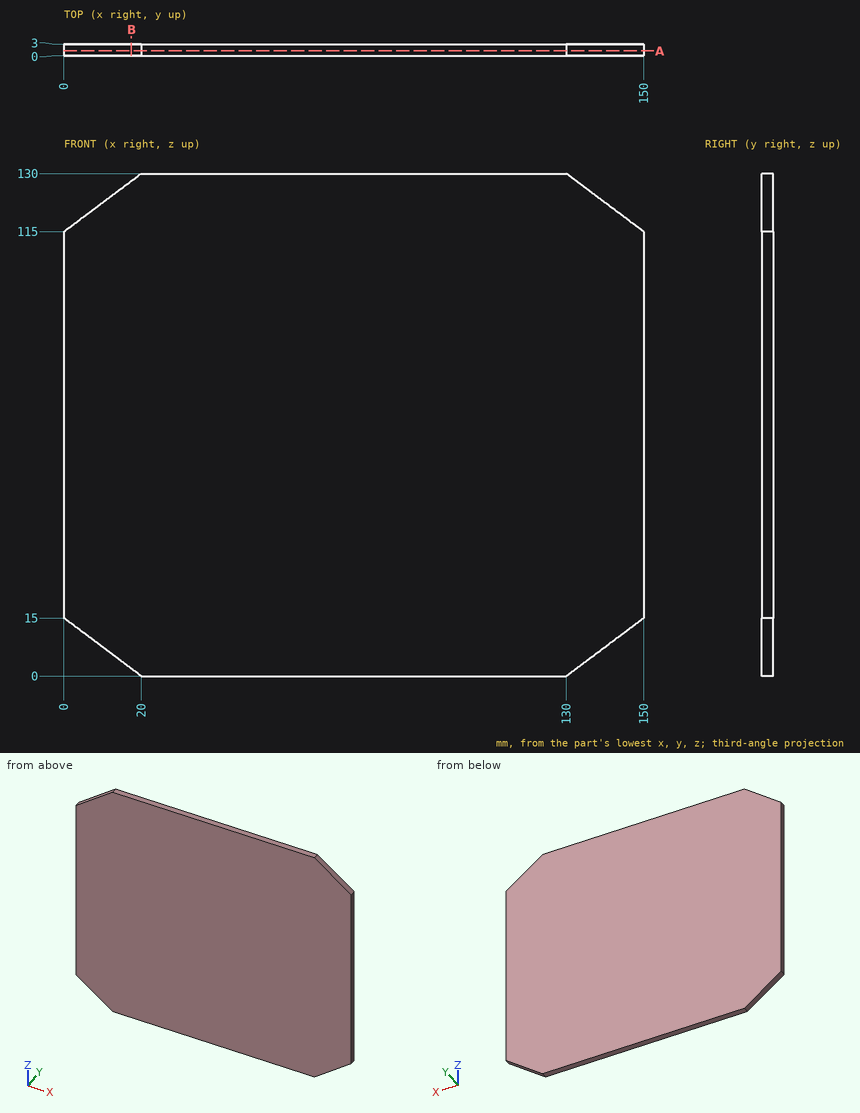
Geometry: see drawing. Coordinates: mm, zero at the bounding-box minimum. Round coordinates to 2 decimals unless told otherwise and drop trailing zeros. Loops run counter-clockwise (first coordinate to the right, second up) from the corner with the lowest first, then second, coordinate; pieces in that order, holes last. Notation, with made-up numbers: (-40, 24) - (19, 24) arc R30 cw to (19, 47) - close; hole circle Ø1 at (59.5, 87). An arc over 180 degrees is marked (long way). Use CSV: the item, a comma, the result in double quotes.
Q1. Section query B-B, the plane x = 17.5. Output: boundary loops of the cut face in (y, z) (3 decimals).
Reported:
outline,"(0, 1.875) - (3, 1.875) - (3, 128.125) - (0, 128.125) - close"
Q2. Section query A-A, the plane y = 1.2. Output: boundary loops of the cut face in (x, z), then the cut area to 3 significant figures.
Reported:
outline,"(0, 15) - (20, 0) - (130, 0) - (150, 15) - (150, 115) - (130, 130) - (20, 130) - (0, 115) - close"
area,"18,900 mm^2"
Q3. Ray query, line 1 along Z through (x, y) = (14, 1.2); line 2 along X through (y, z) = (1.75, 124); line 3 along X through (y, z) = (2.1, 120). Return the intervals inside material, ascending.
Reported:
line 1,"4.5 to 125.5"
line 2,"12 to 138"
line 3,"6.67 to 143.33"
